Read the model definition and answer for the solid it produces. Units are mm, in the model's axes. A direction names the side the tool comes from. Give positions to 0.01 mm unless a question says otherwise; leave off trailing zeros. Order: outer loops, then holes, each group sorted by start corner. A loop starts at its lowest first (then second) coordinate and runs counter-clockwise, first axis right, second up. Notation, with made-up numbers: (49.25, 61.5) - (80.25, 61.5) arc R8 cw to (80.25, 73.5) - close; hole circle Ø5 at (37, -14). An arc over 180 degrees is marked (long way). Write each question's results on one line, items separated by ' | '.
from build123d import *

# Parameters (mm, degrees)
F0_W     = 112.7
F0_H     = 36
F1_DEPTH = 4
F2_R     = 1.35
F3_DEPTH = 4.001
F4_W     = 34
F4_H     = 24
F4_W_2   = 27
F5_DEPTH = 4.001
F6_R     = 4


# Not quite as in the source:
# - a feature names something its author has since deleted; it is built from what else it names


with BuildPart() as f1:
    # F0 (on Top) → F1 (new body)
    with BuildSketch(Plane.XY):
        Rectangle(F0_W, F0_H)
    extrude(amount=F1_DEPTH)

    # F2 (on face) → F3 (cut, through all)
    with BuildSketch(Plane(origin=(0, 0, 0), x_dir=(1, 0, 0), z_dir=(0, 0, -1))):
        with Locations((-53.85, 15)):
            Circle(F2_R)
        with Locations((-53.85, -15)):
            Circle(F2_R)
        with Locations((53.85, 15)):
            Circle(F2_R)
        with Locations((53.85, -15)):
            Circle(F2_R)
    extrude(amount=-F3_DEPTH, mode=Mode.SUBTRACT)

    # F4 (on face) → F5 (cut, through all)
    with BuildSketch(Plane(origin=(0, 0, 0), x_dir=(1, 0, 0), z_dir=(0, 0, -1))):
        with Locations((-33.35, 0)):
            Rectangle(F4_W, F4_H)
        with Locations((3.85, 0)):
            Rectangle(F4_W_2, F4_H)
        with Locations((36.85, 0)):
            Rectangle(F4_W_2, F4_H)
    extrude(amount=-F5_DEPTH, mode=Mode.SUBTRACT)

    # F6
    f6_edges = [f1.edges().sort_by_distance(p)[0] for p in [
        (-16.35, -12, 2),
        (-50.35, -12, 2),
        (-50.35, 12, 2),
        (-16.35, 12, 2),
        (-9.65, -12, 2),
        (23.35, -12, 2),
        (-9.65, 12, 2),
        (17.35, -12, 2),
        (50.35, -12, 2),
        (50.35, 12, 2),
        (23.35, 12, 2),
        (17.35, 12, 2),
    ]]
    fillet(f6_edges, radius=F6_R)


solid = f1.part
(1) This flat-tipped pin is pushed along its axis until it touches: pin 1 (1 mm diameter, centred on x = 21, y = 12.5, fed in from -Z). Where does it stop, or does it pass through?
Conclusion:
pin 1: z = 0
(2) Section B-B (z = 3.25) is taken. State how many separate pieces and enclosed holes the cut face has, plus the area to 3 significant figures.
Conclusion:
separate pieces: 1 | enclosed holes: 7 | area: 1,960 mm^2
(3) Section D-D (x = -53.85) is taken. Give the vertices of the cut face in (y, z).
Conclusion:
outline: (-18, 0) - (-16.35, 0) - (-16.35, 4) - (-18, 4) - close; (-13.65, 0) - (13.65, 0) - (13.65, 4) - (-13.65, 4) - close; (16.35, 0) - (18, 0) - (18, 4) - (16.35, 4) - close
(4) Consider probe 1 along Y at (x, z) = (53.85, 1.5); probe 2 along X at (y, z) = (5, 0.8); probe 3 along X at (y, z) = (-15, 2.15). Determine where each line is inside the solid, lowest interval first. Write a range as [from, to].
Conclusion:
probe 1: [-18, -16.35], [-13.65, 13.65], [16.35, 18] | probe 2: [-56.35, -50.35], [-16.35, -9.65], [17.35, 23.35], [50.35, 56.35] | probe 3: [-56.35, -55.2], [-52.5, 52.5], [55.2, 56.35]
(5) For faces 4 (the face through (-56.35, 0, 2)), 5 (the face through (24.491, 10.797, 2.028)), determine the directions among +Z, -Z, +X, -X, +Y, -Y from which every point of the face is accessible in a straight line to the end or side of a thin tool.
Conclusion:
face 4: +Z, -Z, -X, +Y, -Y | face 5: +Z, -Z
(6) Section A-A (x = 36) is taken. Give the vertices of the cut face in (y, z).
Conclusion:
outline: (-18, 0) - (-12, 0) - (-12, 4) - (-18, 4) - close; (12, 0) - (18, 0) - (18, 4) - (12, 4) - close
(7) Section C-C (y = 15) is taken. Give the vertices of the cut face in (x, z).
Conclusion:
outline: (-56.35, 0) - (-55.2, 0) - (-55.2, 4) - (-56.35, 4) - close; (-52.5, 0) - (52.5, 0) - (52.5, 4) - (-52.5, 4) - close; (55.2, 0) - (56.35, 0) - (56.35, 4) - (55.2, 4) - close
(8) The mould has two halves that part along Y. Classify faces 1 (the face through (-50.35, 0, 2)), 2 (the face through (-13, 0, 4)), 3 (the face through (-1, 18, 2)): pulls with the +Y half, pulls with the -Y half, needs draft (parallel to the pull), parting line crosses it, or undercut.
Conclusion:
face 1: undercut | face 2: needs draft | face 3: pulls with the +Y half
